```python
from build123d import *

# Parameters (mm, degrees)
SKETCH1_R           = 13.5
BOSS_EXTRUDE1_DEPTH = 18.5
SKETCH2_R           = 1.5
BOSS_EXTRUDE2_DEPTH = 3.5
BOSS_EXTRUDE3_START = 3
SKETCH3_R           = 1.5
BOSS_EXTRUDE3_DEPTH = 3
CHAMFER1_SIZE       = 6
CHAMFER2_SIZE       = 2


with BuildPart() as part:
    # Sketch1 → Boss-Extrude1 (new body)
    with BuildSketch(Plane(origin=(0, 0, 0), x_dir=(1, 0, 0), z_dir=(0, 1, 0))):
        with Locations(Location((0, 0, 0), (0, 0, 270))):
            Circle(SKETCH1_R)
    extrude(amount=BOSS_EXTRUDE1_DEPTH)

    # Sketch2 → Boss-Extrude2 (add)
    with BuildSketch(Plane(origin=(0, 18.5, 0), x_dir=(1, 0, 0), z_dir=(0, 1, 0))):
        with Locations(Location((0, 0, 0), (0, 0, 270))):
            Circle(SKETCH2_R)
    extrude(amount=BOSS_EXTRUDE2_DEPTH)

    # Sketch3 → Boss-Extrude3 (add)
    with BuildSketch(Plane.XZ.offset(BOSS_EXTRUDE3_START)):
        with Locations(Location((0, 0, 0), (0, 0, 90))):
            Circle(SKETCH3_R)
    extrude(amount=-BOSS_EXTRUDE3_DEPTH)

    # Chamfer1
    chamfer1_edges = [part.edges().sort_by_distance(p)[0] for p in [
        (0, 18.5, -13.5),
    ]]
    chamfer(chamfer1_edges, length=CHAMFER1_SIZE)

    # Chamfer2
    chamfer2_edges = [part.edges().sort_by_distance(p)[0] for p in [
        (0, 0, -13.5),
    ]]
    chamfer(chamfer2_edges, length=CHAMFER2_SIZE)


solid = part.part
```
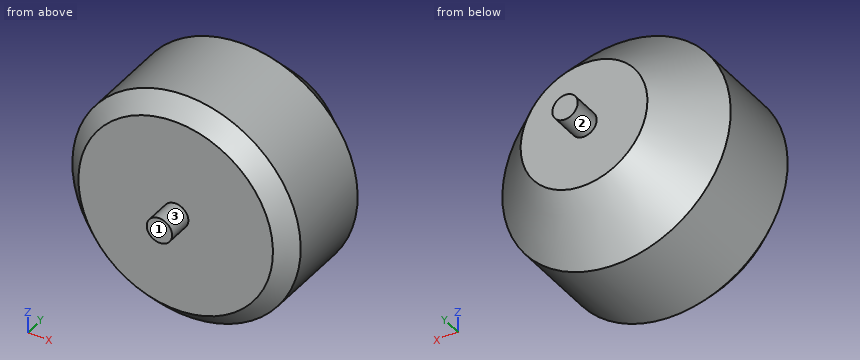
Model file for the job. Use its own axes, mm. Face numbers are marked on the shaded views. A direction names the side the tool comes from. Coordinates: 2 decimals unless noted, no trailing zeros. Order: outer loops, then holes, each group sorted by start corner. A loop starts at its lowest first (then second) coordinate and runs counter-clockwise, first axis right, second up. Notation, with made-up numbers: (77.5, -23.75) -> (83.5, -23.75) arc R25 cw to (83.5, -0.75) -> close; hole circle Ø3 at (-34.5, 46.5). An arc over 180 degrees is marked (long way). Answer as a JSON object with one key per item and string values. Group by question number.
1) Cut at B-B, the plane z = 0. Write the cut outline in (x, y), then the cut area to 3 significant figures.
2) Drill centre lines: L1, parallel to Y at x = 2, z = -3.5; L2, parallel to X at y = 17.5, z = 0.75; L3, parallel to Z at x = -12.5, y = 4.75. Where is each one in solid material? Low to high.
3) Cut at C-C, the plane y = 19.75. Write the cut outline in (x, z), then the cut area to 3 significant figures.
4) Which spindle directions (+Z, -Z, +X, -X, +Y, -Y) get a long thin tool onto all of the face, cutting with end or side? Do the marked faces 1, 2 and 3. Say none if no direction does.
5) Cut at A-A, the plane x = 0. Write the cut outline in (y, z).
6) Cut at D-D, the plane y = 3.5. Write the cut outline in (x, z).
7) Flat gauge pins, fed straight in: pin 1 (8 mm diameter, centred on x = 7, y = 12, fed in from -Z); pin 2 (8 mm diameter, centred on y = 13.5, z = -4.5, fed in from +X); pin 3 (10 mm diameter, centred on x = 6, z = -10, fed in from -Y); pin 4 (10 mm diameter, centred on x = -2, y = 8.5, fed in from +Z). Where does each tip first touch, or does it go through?
Check values:
{
 "1": {"outline": "(-13.5, 2) -> (-11.5, 0) -> (-1.5, 0) -> (-1.5, -3) -> (1.5, -3) -> (1.5, 0) -> (11.5, 0) -> (13.5, 2) -> (13.5, 12.5) -> (7.5, 18.5) -> (1.5, 18.5) -> (1.5, 22) -> (-1.5, 22) -> (-1.5, 18.5) -> (-7.5, 18.5) -> (-13.5, 12.5) -> close", "area": "479 mm²"},
 "2": {"L1": "y = 0 to 18.5", "L2": "x = -8.47 to 8.47", "L3": "z = -5.1 to 5.1"},
 "3": {"outline": "circle Ø3 at (0, 0)", "area": "7.07 mm²"},
 "4": {"face 1": "+Z, -Z, +X, -X, -Y", "face 2": "+Y", "face 3": "-Y"},
 "5": {"outline": "(-3, -1.5) -> (0, -1.5) -> (0, -11.5) -> (2, -13.5) -> (12.5, -13.5) -> (18.5, -7.5) -> (18.5, -1.5) -> (22, -1.5) -> (22, 1.5) -> (18.5, 1.5) -> (18.5, 7.5) -> (12.5, 13.5) -> (2, 13.5) -> (0, 11.5) -> (0, 1.5) -> (-3, 1.5) -> close"},
 "6": {"outline": "circle Ø27 at (0, 0)"},
 "7": {"pin 1": "stops at z = -13.16", "pin 2": "stops at x = 13.49", "pin 3": "stops at y = 0", "pin 4": "stops at z = 13.5"}
}
